Source: CAD feature listing. Evaluate the final solid. Frame: model axes, mm. Round coordinates to 2 decimals unless told otherwise and drop trailing zeros. Write each loop counter-clockwise with the first axis right and the second up, starting at its lowest first coordinate (ties: lowest second). Pieces come first, ordered by that corner, then holes. Notation, with made-up numbers: M 34,18.25 L 52,18.25 A20 cw 52,45.25 Z; hole C -8,-30.75 d6. An arc over 180 degrees is marked long. Answer in a Markdown table with one row per item. Add a question column.
Item 1: Cut plane B-B on y = 1.7. Give the number of separate pieces and of enclosed holes in the cut face, and give its area (3 significant figures).
Item 2: Cut plane A-A on z = 38. Return loops of the section in (x, y), and give its area (3 significant figures).
Item 3: Mould query, pull axis X, two halves, no side actions, for faces 1 (the face through (121.99, 1.52, 67.15)), 2 (the face through (14.504, 1.479, 9.228)), 3 (the face through (0.676, 1.479, -6.164)), 4 (the face through (-2, 3, -1)). Classes: released by +X, released by -X, zero draft, split by the parting line, or undercut.
Item 4: Contact query for a flat-ended pin moving along its axis: pin 1 (3 mm diameter, centred on x = 96, z = 0, fed in from +Y). Output: stop coordinate, or through.
Item 5: Material intervals for probe 1 along Z at (x, y) = (-115, 2.1); probe 2 along X at (y, z) = (1.3, -33); probe 3 along Z at (x, y) = (25, 1.55), sorted ascending.
from build123d import *

# Parameters (mm, degrees)
SKETCH1_W               = 250
SKETCH1_H               = 140
BOSS_EXTRUDE1_DEPTH     = 3
FILLET2_R               = 10
CUT_EXTRUDE5_DEPTH      = 7
CUT_EXTRUDE5_DEPTH_BACK = 7
SKETCH2_R               = 1.6
SKETCH2_R_2             = 1.4
SKETCH2_R_3             = 2.25
SKETCH2_R_4             = 1.55
CUT_EXTRUDE6_DEPTH      = 7
CUT_EXTRUDE6_DEPTH_BACK = 7
SKETCH3_R               = 1.6
CUT_EXTRUDE7_DEPTH      = 7
CUT_EXTRUDE7_DEPTH_BACK = 7
SKETCH4_R               = 1.6
CUT_EXTRUDE8_DEPTH      = 7
CUT_EXTRUDE8_DEPTH_BACK = 7
SKETCH5_R               = 1.4
SKETCH5_W               = 11.7
SKETCH5_H               = 18.9
SKETCH5_R_2             = 3.4
SKETCH5_R_3             = 6.2
CUT_EXTRUDE9_DEPTH      = 144.296894593
CUT_EXTRUDE9_DEPTH_BACK = 144.296894593
SKETCH6_R               = 1.6


with BuildPart() as part:
    # Sketch1 → Boss-Extrude1 (new body)
    with BuildSketch(Plane(origin=(0, 0, 0), x_dir=(1, 0, 0), z_dir=(0, 1, 0))):
        Rectangle(SKETCH1_W, SKETCH1_H)
    extrude(amount=BOSS_EXTRUDE1_DEPTH)

    # Fillet2
    fillet2_edges = [part.edges().sort_by_distance(p)[0] for p in [
        (125, 1.5, 70),
        (-125, 1.5, 70),
        (-125, 1.5, -70),
        (125, 1.5, -70),
    ]]
    fillet(fillet2_edges, radius=FILLET2_R)

    # Sketch2 → Cut-Extrude5 (cut, two sides: drawn at the far end of the back side and taken through both)
    with BuildSketch(Plane(origin=(0, 0, 0), x_dir=(1, 0, 0), z_dir=(0, 1, 0)).offset(-CUT_EXTRUDE5_DEPTH_BACK)):
        with Locations(Location((-104, 0, 0), (0, 0, 270))):
            Circle(SKETCH2_R)
        with Locations(Location((-57, 46, 0), (0, 0, 270))):
            Circle(SKETCH2_R_2)
        with Locations(Location((-57, -46, 0), (0, 0, 270))):
            Circle(SKETCH2_R_2)
        with Locations(Location((-115, -46, 0), (0, 0, 270))):
            Circle(SKETCH2_R_2)
        with Locations(Location((-115, 46, 0), (0, 0, 270))):
            Circle(SKETCH2_R_2)
        with Locations(Location((-16.5, -8.189424071, 0), (0, 0, 270))):
            Circle(SKETCH2_R_3)
        with Locations(Location((0, 8.310575929, 0), (0, 0, 270))):
            Circle(SKETCH2_R_3)
        with Locations(Location((16.5, -8.189424071, 0), (0, 0, 270))):
            Circle(SKETCH2_R_3)
        with Locations(Location((37, 0.060575929, 0), (0, 0, 270))):
            Circle(SKETCH2_R_3)
        with Locations(Location((20.5, -16.439424071, 0), (0, 0, 270))):
            Circle(SKETCH2_R_3)
        with Locations(Location((-13, -18.939424071, 0), (0, 0, 270))):
            Circle(SKETCH2_R)
        with Locations(Location((40, -18.939424071, 0), (0, 0, 270))):
            Circle(SKETCH2_R)
        with Locations(Location((20.5, 16.560575929, 0), (0, 0, 270))):
            Circle(SKETCH2_R_3)
        with Locations(Location((-13, -55.939424071, 0), (0, 0, 270))):
            Circle(SKETCH2_R)
        with Locations(Location((40, -55.939424071, 0), (0, 0, 270))):
            Circle(SKETCH2_R)
        with Locations(Location((96, 0, 0), (0, 0, 270))):
            Circle(SKETCH2_R)
        with Locations(Location((68, 18, 0), (0, 0, 270))):
            Circle(SKETCH2_R_4)
        with Locations(Location((68, -18, 0), (0, 0, 270))):
            Circle(SKETCH2_R_4)
        with Locations(Location((116, 18, 0), (0, 0, 270))):
            Circle(SKETCH2_R_4)
        with Locations(Location((116, -18, 0), (0, 0, 270))):
            Circle(SKETCH2_R_4)
    extrude(amount=CUT_EXTRUDE5_DEPTH + CUT_EXTRUDE5_DEPTH_BACK, mode=Mode.SUBTRACT)

    # Sketch3 → Cut-Extrude6 (cut, two sides: drawn at the far end of the back side and taken through both)
    with BuildSketch(Plane(origin=(0, 0, 0), x_dir=(1, 0, 0), z_dir=(0, 1, 0)).offset(-CUT_EXTRUDE6_DEPTH_BACK)):
        with Locations(Location((-96.745, -32.704968659, 0), (0, 0, 270))):
            Circle(SKETCH3_R)
    extrude(amount=CUT_EXTRUDE6_DEPTH + CUT_EXTRUDE6_DEPTH_BACK, mode=Mode.SUBTRACT)

    # Sketch4 → Cut-Extrude7 (cut, two sides: drawn at the far end of the back side and taken through both)
    with BuildSketch(Plane(origin=(0, 3, 0), x_dir=(1, 0, 0), z_dir=(0, 1, 0)).offset(-CUT_EXTRUDE7_DEPTH_BACK)):
        with Locations(Location((90.54, -34.065208057, 0), (0, 0, 270))):
            Circle(SKETCH4_R)
        with Locations(Location((90.54, 34.065208057, 0), (0, 0, 270))):
            Circle(SKETCH4_R)
    extrude(amount=CUT_EXTRUDE7_DEPTH + CUT_EXTRUDE7_DEPTH_BACK, mode=Mode.SUBTRACT)

    # Sketch5 → Cut-Extrude8 (cut, two sides: drawn at the far end of the back side and taken through both)
    with BuildSketch(Plane(origin=(0, 3, 0), x_dir=(1, 0, 0), z_dir=(0, 1, 0)).offset(-CUT_EXTRUDE8_DEPTH_BACK)):
        with Locations(Location((102, -31.945997938, 0), (0, 0, 270))):
            Circle(SKETCH5_R)
        with Locations((102, -44.445997938)):
            Rectangle(SKETCH5_W, SKETCH5_H)
        with Locations(Location((102, -56.945997938, 0), (0, 0, 270))):
            Circle(SKETCH5_R)
        with Locations(Location((-110, -60, 0), (0, 0, 270))):
            Circle(SKETCH5_R_2)
        Polygon((-54, -56), (-54, -60), (-54, -64), (-46, -64), (-46, -56), align=None)
        with Locations(Location((-80, -60, 0), (0, 0, 270))):
            Circle(SKETCH5_R_3)
        with Locations(Location((-110, 60, 0), (0, 0, 270))):
            Circle(SKETCH5_R_2)
        Polygon((0, 47.5), (-27.5, 47.5), (-27.5, 32.5), (27.5, 32.5), (27.5, 47.5), align=None)
    extrude(amount=CUT_EXTRUDE8_DEPTH + CUT_EXTRUDE8_DEPTH_BACK, mode=Mode.SUBTRACT)

    # Sketch6 → Cut-Extrude9 (cut, two sides: drawn at the far end of the back side and taken through both)
    with BuildSketch(Plane(origin=(0, 3, 0), x_dir=(1, 0, 0), z_dir=(0, 1, 0)).offset(-CUT_EXTRUDE9_DEPTH_BACK)):
        with Locations(Location((-17.5, 59.5, 0), (0, 0, 270))):
            Circle(SKETCH6_R)
        with Locations(Location((47.5, 59.5, 0), (0, 0, 270))):
            Circle(SKETCH6_R)
        with Locations(Location((-17.5, 20.5, 0), (0, 0, 270))):
            Circle(SKETCH6_R)
        with Locations(Location((47.5, 20.5, 0), (0, 0, 270))):
            Circle(SKETCH6_R)
    extrude(amount=CUT_EXTRUDE9_DEPTH + CUT_EXTRUDE9_DEPTH_BACK, mode=Mode.SUBTRACT)


solid = part.part
Results below:
| question | item | result |
|---|---|---|
| 1 | separate pieces | 1 |
| 1 | enclosed holes | 35 |
| 1 | area | 33,300 mm2 |
| 2 | outline | M -125,0 L 96.15,0 L 96.15,3 L -125,3 Z; M 107.85,0 L 125,0 L 125,3 L 107.85,3 Z |
| 2 | area | 715 mm2 |
| 3 | face 1 | released by +X |
| 3 | face 2 | undercut |
| 3 | face 3 | undercut |
| 3 | face 4 | zero draft |
| 4 | pin 1 | through |
| 5 | probe 1 | -70 to -47.4, -44.6 to 44.6, 47.4 to 70 |
| 5 | probe 2 | -125 to -27.5, 27.5 to 89.35, 91.73 to 125 |
| 5 | probe 3 | -70 to -47.5, -32.5 to 70 |
